Autodesk Inventor part; units mm, degrees
ref_plane "YZ Plane" through (0, 0, 0) normal (1, 0, 0) x (0, 1, 0)
ref_plane "XZ Plane" through (0, 0, 0) normal (0, 1, 0) x (-1, 0, 0)
ref_plane "XY Plane" through (0, 0, 0) normal (0, 0, 1) x (1, 0, 0)
sketch "스케치3" plane through (0, 0, 0) normal (0, 1, 0) x (-1, 0, 0)
  line L0 (34.9919, -14.4941) -> (14.4941, -34.9919)
  line L1 (14.4941, -34.9919) -> (-14.4941, -34.9919)
  line L2 (-14.4941, -34.9919) -> (-34.9919, -14.4941)
  line L3 (-34.9919, -14.4941) -> (-34.9919, 14.4941)
  line L4 (-34.9919, 14.4941) -> (-14.4941, 34.9919)
  line L5 (-14.4941, 34.9919) -> (14.4941, 34.9919)
  line L6 (14.4941, 34.9919) -> (34.9919, 14.4941)
  line L7 (34.9919, 14.4941) -> (34.9919, -14.4941)
  line L8 (32.5919, -13.5) -> (13.5, -32.5919)
  line L9 (13.5, -32.5919) -> (-13.5, -32.5919)
  line L10 (-13.5, -32.5919) -> (-32.5919, -13.5)
  line L11 (-32.5919, -13.5) -> (-32.5919, 13.5)
  line L12 (-32.5919, 13.5) -> (-13.5, 32.5919)
  line L13 (-13.5, 32.5919) -> (13.5, 32.5919)
  line L14 (13.5, 32.5919) -> (32.5919, 13.5)
  line L15 (32.5919, 13.5) -> (32.5919, -13.5)
  point P0 (0, 0)
  point P1 (0, 0)
  point P2 (0, 0)
  point P3 (0, 0)
  dimension "d43" = 27
  dimension "d44" = 2.4
extrude "돌출2" add sketch "스케치3" along normal blind 3.4 contours L0 L1 L2 L3 L4 L5 L6 L7 | L8 L9 L10 L11 L12 L13 L14 L15
sketch "스케치4" plane through (0, 3.4, 0) normal (0, 1, 0) x (1, 0, 0)
  line L0 (13.5, -32.5919) -> (-13.5, -32.5919)
  line L1 (-13.5, -32.5919) -> (-32.5919, -13.5)
  line L2 (-32.5919, -13.5) -> (-32.5919, 13.5)
  line L3 (-32.5919, 13.5) -> (-13.5, 32.5919)
  line L4 (-13.5, 32.5919) -> (13.5, 32.5919)
  line L5 (13.5, 32.5919) -> (32.5919, 13.5)
  line L6 (32.5919, 13.5) -> (32.5919, -13.5)
  line L7 (32.5919, -13.5) -> (13.5, -32.5919)
  line L8 (-13.9971, 33.7919) -> (13.9971, 33.7919)
  line L9 (13.9971, 33.7919) -> (33.7919, 13.9971)
  line L10 (33.7919, 13.9971) -> (33.7919, -13.9971)
  line L11 (33.7919, -13.9971) -> (13.9971, -33.7919)
  line L12 (13.9971, -33.7919) -> (-13.9971, -33.7919)
  line L13 (-13.9971, -33.7919) -> (-33.7919, -13.9971)
  line L14 (-33.7919, -13.9971) -> (-33.7919, 13.9971)
  line L15 (-33.7919, 13.9971) -> (-13.9971, 33.7919)
  line L16 (-13.1686, 31.7919) -> (13.1686, 31.7919)
  line L17 (13.1686, 31.7919) -> (31.7919, 13.1686)
  line L18 (31.7919, 13.1686) -> (31.7919, -13.1686)
  line L19 (31.7919, -13.1686) -> (13.1686, -31.7919)
  line L20 (13.1686, -31.7919) -> (-13.1686, -31.7919)
  line L21 (-13.1686, -31.7919) -> (-31.7919, -13.1686)
  line L22 (-31.7919, -13.1686) -> (-31.7919, 13.1686)
  line L23 (-31.7919, 13.1686) -> (-13.1686, 31.7919)
  point P0 (0, 0)
  point P1 (0, 0)
  point P2 (0, 0)
  point P3 (0, 0)
  dimension "d7" = 27
  dimension "d42" = 1.2
  dimension "d45" = 0.8
extrude "돌출3" cut sketch "스케치4" against normal blind 0.8 contours L0 L1 L2 L3 L4 L5 L6 L7 | L8 L9 L10 L11 L12 L13 L14 L15
sketch "스케치5" plane through (0, 0, 0) normal (0, -1, 0) x (1, 0, 0)
  line L0 (10, 2.5) -> (20, 2.5)
  line L1 (20, 2.5) -> (20, -2.5)
  line L2 (20, -2.5) -> (10, -2.5)
  line L3 (10, -2.5) -> (10, 2.5)
  line L4 (10, 2.5) -> (20, -2.5) construction
  line L5 (20, 2.5) -> (10, -2.5) construction
  line L6 (-20, 2.5) -> (-10, 2.5)
  line L7 (-10, 2.5) -> (-10, -2.5)
  line L8 (-10, -2.5) -> (-20, -2.5)
  line L9 (-20, -2.5) -> (-20, 2.5)
  line L10 (-20, 2.5) -> (-10, -2.5) construction
  line L11 (-10, 2.5) -> (-20, -2.5) construction
  point P0 (0, 0)
  point P1 (15, 0)
  point P2 (-15, 0)
  dimension "d11" = 10
  dimension "d12" = 5
  dimension "d13" = 10
  dimension "d16" = 30
extrude "돌출4" add sketch "스케치5" along normal blind 10
sketch "스케치6" plane through (-10, 0, -2.5) normal (0, 0, -1) x (-1, 0, 0)
  circle A0 centre (5, -10) radius 5
  circle A1 centre (-25, -10) radius 5
  line L0 (-20, -10) -> (-30, -10)
  line L1 (10, -10) -> (0, -10)
  point P0 (-10, 0)
  dimension "d23" = 10
  dimension "d24" = 10
extrude "돌출5" add sketch "스케치6" against normal blind 5
sketch "스케치7" plane through (-10, 0, -2.5) normal (0, 0, -1) x (-1, 0, 0)
  circle A0 centre (5, -10) radius 1.25
  line L0 (10, 0) -> (10, -10)
  line L1 (0, 0) -> (10, 0)
  line L2 (4.7788, 0) -> (0, 0)
  circle A1 centre (-25, -10) radius 1.25
  point P0 (-10, 0)
  dimension "d27" = 2.5
  dimension "d28" = 5
  dimension "d31" = 30
extrude "돌출6" cut sketch "스케치7" against normal blind 5
sketch "스케치8" plane through (0, 0, 0) normal (0, -1, 0) x (1, 0, 0)
  circle A0 centre (0, -17.3205) radius 1.25
  line L0 (-10, 2.5) -> (-10, -2.5)
  point P0 (0, 0)
  point P1 (-10, 0)
  dimension "d38" = 2.5
  dimension "d39" = 17.3205
extrude "돌출7" cut sketch "스케치8" against normal blind 5
properties part number "팔각형 OV-PAM 5패턴 상단 - 틈 너비 수정"
Geometry check sheet. Reference: the model listing, model coordinates, mm. A direction names the side the tool comes from. Coordinates: 2 decimals unless noted, no trailing zeros. Order: outer loops, then holes, each group sorted by start corner. A loop starts at its lowest first (then second) coordinate and runs counter-clockwise, first axis right, second up. Notation, with made-up numbers: (-13, 75.25) - (45, 75.25) arc R18 cw to (45, 105.25) - close; hole circle Ø6 at (-33.75, 16). An arc over 180 degrees is marked (long way). One line per item, written item: value.
(1) Thickness scan on probe 1 along Y at (x, z) = (15, 0); probe 2 along Z at (x, y) = (0, 0.85); probe 3 along Y at (x, z) = (2.5, -30). Record the ranges inside material, lowest first. Write a range as from..to.
Data:
probe 1: y = -15..-11.25, -8.75..3.4
probe 2: z = -34.99..-18.57, -16.07..34.99
probe 3: y = 0..3.4
(2) Sectioned sample at A-A (x = 0). Enter the section's corners in (y, z).
Data:
outline: (0, -34.99) - (3.4, -34.99) - (3.4, -33.79) - (2.6, -33.79) - (2.6, -31.79) - (3.4, -31.79) - (3.4, -18.57) - (0, -18.57) - close; (0, -16.07) - (3.4, -16.07) - (3.4, 31.79) - (2.6, 31.79) - (2.6, 33.79) - (3.4, 33.79) - (3.4, 34.99) - (0, 34.99) - close
(3) Sectioned sample at C-C (z = 9). Enter the section's corners in (x, y), and give its area (3 significant figures).
Data:
outline: (-34.99, 0) - (34.99, 0) - (34.99, 3.4) - (33.79, 3.4) - (33.79, 2.6) - (31.79, 2.6) - (31.79, 3.4) - (-31.79, 3.4) - (-31.79, 2.6) - (-33.79, 2.6) - (-33.79, 3.4) - (-34.99, 3.4) - close
area: 235 mm^2
(4) Sectioned sample at D-D (x = 18). Enter the section's corners in (y, z).
Data:
outline: (-14, -2.5) - (0, -2.5) - (0, -31.49) - (3.4, -31.49) - (3.4, -29.79) - (2.6, -29.79) - (2.6, -26.96) - (3.4, -26.96) - (3.4, 26.96) - (2.6, 26.96) - (2.6, 29.79) - (3.4, 29.79) - (3.4, 31.49) - (0, 31.49) - (0, 2.5) - (-14, 2.5) - close
(5) Depth check by flat-ended pin: pin 1 Ø2.5 at (y, z) = (-4.5, 1) entering from +X; pin 2 Ø1 at (y, z) = (-9, 2.5) entering from -X; pin 3 Ø8 at (x, z) = (3, 12.5) entering from -Y; pin 4 Ø2 at (x, y) = (15, -10) entering from -Z. Enter the tip coordinate at first touch or a pass-through.
Data:
pin 1: stops at x = 20
pin 2: stops at x = -20
pin 3: stops at y = 0
pin 4: passes through
(6) Release check for a two-part mould opening along X. For faces 1 (the face through (15, -7, -2.5)), 2 (the face through (-24.886, 1.676, -24.6)), 3 (the face through (-23.76, 3.01, 24.03)) record: +X half, -X half, draft (parallel to the pull), parting line (faces both ways), or undercut.
Data:
face 1: draft
face 2: -X half
face 3: undercut
(7) Sectioned sample at B-B (y = -4.25). Enter the section's corners in (x, z), and give its area (3 significant figures).
Data:
outline: (-20, -2.5) - (-10, -2.5) - (-10, 2.5) - (-20, 2.5) - close; (10, -2.5) - (20, -2.5) - (20, 2.5) - (10, 2.5) - close
area: 100 mm^2
(8) Access from +Z, -Z, +X, -X, +Y, -Y to the whole of each face (thin tool, end or side, straight path). Record for faces 4 (the face through (22.35, 3.01, -22.61)), 5 (the face through (-10, -5, 0)), 6 (the face through (20, -5, 0)), 7 (the face through (15, -7, 2.5)).
Data:
face 4: +Y
face 5: +Z, -Z, -Y
face 6: +Z, -Z, +X, -Y
face 7: +Z, +X, -X, -Y
